Work out the finished part from the listing and answer in its coordinate system (mm). A direction names the side the tool comes from. Give positions to 0.01 mm unless a question says otherwise; leave off trailing zeros. Loops run counter-clockwise (first coordinate to the right, second up) from the corner with the lowest first, then second, coordinate; pieces in that order, holes last. Notation, with made-up numbers: (16, 54) - (41, 54) arc R19 cw to (41, 73) - close; hole circle Ø6 at (57.5, -5). An arc over 180 degrees is marked (long way). Use one line per item in the form item = value. Start each with the question number.
from build123d import *

# Parameters (mm, degrees)
BOSS_EXTRUDE1_DEPTH = 55
CUT_EXTRUDE1_DEPTH  = 80


with BuildPart() as part:
    # Sketch1 → Boss-Extrude1 (new body, symmetric)
    with BuildSketch(Plane(origin=(0, 0, 0), x_dir=(1, 0, 0), z_dir=(0, 1, 0))):
        with BuildLine():
            Line((-24.819347292, -3), (-21.794494718, -3))
            ThreePointArc((-21.794494718, -3), (0, -22), (21.794494718, -3))
            Line((21.794494718, -3), (24.819347292, -3))
            ThreePointArc((24.819347292, -3), (0, -25), (-24.819347292, -3))
        make_face()
    extrude(amount=BOSS_EXTRUDE1_DEPTH, both=True)

    # Sketch2 → Cut-Extrude1 (cut)
    with BuildSketch(Plane.XY):
        with BuildLine():
            Line((-10, -20), (-10, 20))
            ThreePointArc((-10, 20), (0, 30), (10, 20))
            Line((10, 20), (10, -20))
            ThreePointArc((10, -20), (0, -30), (-10, -20))
        make_face()
    extrude(amount=CUT_EXTRUDE1_DEPTH, mode=Mode.SUBTRACT)


solid = part.part
1) A cutting plane is placed at D-D (x = -11). Give the vertices of the cut face in (y, z).
2) A cutting plane is placed at A-A (y = -12). Give the vertices of the cut face in (x, z), plus the area to 3 significant figures.
3) Find the intervals of material crossed by probe 1 along X at (y, z) = (-32.5, 13.5); probe 2 along X at (y, z) = (-21.5, 9.75); probe 3 along Z at (x, y) = (-10, -50), in increasing order.
4) Flat-ended cylindrical pins translate along their axes: pin 1 Ø10 at (y, z) = (-43, 6) entering from +X; pin 2 Ø1.7 at (y, z) = (-2.5, 20.5) entering from -X; pin 3 Ø4 at (x, y) = (-3, -38) entering from +Z; pin 4 Ø3.5 at (y, z) = (8.5, 20.5) entering from +X. Find the tip coordinate at first contact, or state that the pin passes through.
5) A cutting plane is placed at B-B (z = 9.5). Give the vertices of the cut face in (x, y).
6) A cutting plane is placed at C-C (y = -45). Give the vertices of the cut face in (x, z), plus the area to 3 significant figures.
7) A tool of negligible diameter and unlimited length cuts with its end or side. For faces 1 (the cylindrical face through (-0.2, 30, 22.3)), 2 (the cylindrical face through (-13.444, 0.77, 17.415)), from which of +Z, -Z, +X, -X, +Y, -Y can it reach the whole face along a straight path? Write none if from no direction.
8) Determine the mould class of faces 3 (the flat face through (-10, 0, 21)), 4 (the flat face through (-1.7, 55, 22.1)), 5 (the flat face through (-1.7, -55, 22.1)), 6 (the flat face through (23, 1, 3)) for opening direction Y: released by +Y, released by -Y, zero draft, split by the parting line, or undercut.
Answer sheet:
q1.outline = (-55, 19.05) - (55, 19.05) - (55, 22.45) - (-55, 22.45) - close
q2.outline = (-24.82, 3) - (-21.79, 3) arc R22 cw to (-10, 19.6) - (-10, 22.91) arc R25 ccw to start; (10, 19.6) arc R22 cw to (21.79, 3) - (24.82, 3) arc R25 ccw to (10, 22.91) - close
q2.area = 141 mm²
q3.probe_1 = -21.04 to -17.37, 17.37 to 21.04
q3.probe_2 = -23.02 to -19.72, 19.72 to 23.02
q3.probe_3 = 19.6 to 22.91
q4.pin_1 = 24.82
q4.pin_2 = -15.46
q4.pin_3 = 24.98
q4.pin_4 = 16.54
q5.outline = (-23.12, -55) - (-19.84, -55) - (-19.84, 55) - (-23.12, 55) - close; (19.84, -55) - (23.12, -55) - (23.12, 55) - (19.84, 55) - close
q6.outline = (-24.82, 3) - (-21.79, 3) arc R22 cw to (21.79, 3) - (24.82, 3) arc R25 ccw to start
q6.area = 203 mm²
q7.face_1 = +Z, -Z
q7.face_2 = -Z, +Y, -Y
q8.face_3 = undercut
q8.face_4 = released by +Y
q8.face_5 = released by -Y
q8.face_6 = zero draft
